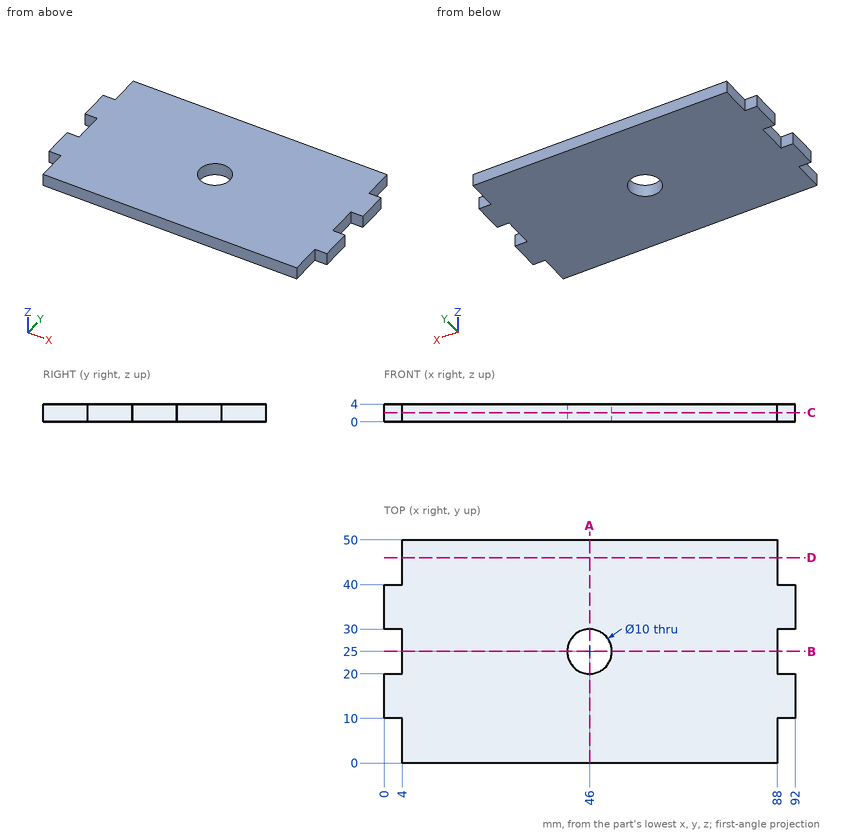
The drawing under review shows one solid part. Ordinate dimensions are in mm from its lowest x, y, z. Give positions to 0.01 mm unless a question says otherwise; leave off trailing zeros. Loops run counter-clockwise (first coordinate to the right, second up) from the corner with the lowest first, then second, coordinate; pieces in that order, holes last. Notation, with made-up numbers: M 40.5,20.5 L 56.5,20.5 A35 cw 56.5,56.5 Z; hole C 83.25,86 d8. An arc over 180 degrees is marked long. Return JSON: item names as keys, results as strings. Group by question number.
Item 1: For probe 1 along Y at (x, z) = (46, 0.8); probe 2 along X at (y, z) = (26, 0.65); probe 3 along X at (y, z) = (3.5, 1.95), list the stretches that pass through material, from the lowest coordinate up.
Item 2: We need section B-B (y = 25). Give the boundary of the cut face in (x, z), and give its area (3 significant figures).
Item 3: We need section A-A (x = 46). Give the boundary of the cut face in (y, z), and give its area (3 significant figures).
Item 4: Insertion check: pin 1 Ø1.2 at (y, z) = (25.5, 1.5) entering from +X; pin 2 Ø1.2 at (x, z) = (3, 2.5) entering from -Y; pin 3 Ø1.2 at (y, z) = (24.5, 2.5) entering from -X. Each pin has a flat end and moves straight along its axis. Give the tip position at first contact, or say it passes through.
Item 5: We need section C-C (z = 2.05). Give the boundary of the cut face in (x, y), and give its area (3 significant figures).
Item 6: We need section D-D (y = 46). Give the boundary of the cut face in (x, z).
Output:
{
 "1": {"probe 1": "y = 0 to 20, 30 to 50", "probe 2": "x = 4 to 41.1, 50.9 to 88", "probe 3": "x = 4 to 88"},
 "2": {"outline": "M 4,0 L 41,0 L 41,4 L 4,4 Z; M 51,0 L 88,0 L 88,4 L 51,4 Z", "area": "296 mm^2"},
 "3": {"outline": "M 0,0 L 20,0 L 20,4 L 0,4 Z; M 30,0 L 50,0 L 50,4 L 30,4 Z", "area": "160 mm^2"},
 "4": {"pin 1": "stops at x = 88", "pin 2": "stops at y = 10", "pin 3": "stops at x = 4"},
 "5": {"outline": "M 0,10 L 4,10 L 4,0 L 88,0 L 88,10 L 92,10 L 92,20 L 88,20 L 88,30 L 92,30 L 92,40 L 88,40 L 88,50 L 4,50 L 4,40 L 0,40 L 0,30 L 4,30 L 4,20 L 0,20 Z; hole C 46,25 d10", "area": "4,280 mm^2"},
 "6": {"outline": "M 4,0 L 88,0 L 88,4 L 4,4 Z"}
}
